Model file for the job. Use its own axes, mm. A direction names the side the tool comes from. Round coordinates to 2 decimals unless told otherwise and drop trailing zeros. Write each loop counter-clockwise with the first axis right and the second up, starting at its lowest first coordinate (ties: lowest second). Pieces come first, ordered by that corner, then holes. Notation, with made-up numbers: (-5.75, 68) - (22.25, 68) arc R35 cw to (22.25, 107) - close; hole circle Ø4 at (20.5, -4). An arc over 180 degrees is marked (long way). Answer as a JSON object with one key per item and string values. Group by question number.
Autodesk Inventor part; units mm, degrees
ref_plane "YZ Plane" through (0, 0, 0) normal (1, 0, 0) x (0, 1, 0)
ref_plane "XZ Plane" through (0, 0, 0) normal (0, 1, 0) x (-1, 0, 0)
ref_plane "XY Plane" through (0, 0, 0) normal (0, 0, 1) x (1, 0, 0)
sketch "Sketch1" plane through (0, 0, 0) normal (0, 1, 0) x (-1, 0, 0)
  line L0 (32, 55) -> (-32, 55)
  line L1 (-32, 55) -> (-32, -55)
  line L2 (-32, -55) -> (32, -55)
  line L3 (32, -55) -> (32, 55)
  line L4 (32, 55) -> (-32, -55) construction
  line L5 (-32, 55) -> (32, -55) construction
  point P0 (0, 0)
  dimension "d0" = 64
  dimension "d1" = 110
extrude "Extrusion1" add sketch "Sketch1" along normal blind 3
sketch "Sketch2" plane through (0, 3, 0) normal (0, 1, 0) x (1, 0, 0)
  line L0 (-32, -55) -> (32, -55)
  line L1 (32, -55) -> (32, 55)
  line L2 (32, 55) -> (-32, 55)
  line L3 (-32, 55) -> (-32, -55)
  line L4 (-32, -55) -> (32, -55)
  line L5 (32, -55) -> (32, 55)
  line L6 (32, 55) -> (-32, 55)
  line L7 (-32, 55) -> (-32, -55)
  line L8 (-32, -55) -> (32, 55) construction
  line L9 (32, -55) -> (-32, 55) construction
  line L10 (-29, -52) -> (29, -52)
  line L11 (29, -52) -> (29, 52)
  line L12 (29, 52) -> (-29, 52)
  line L13 (-29, 52) -> (-29, -52)
  point P0 (0, 0)
  dimension "d4" = 3
  dimension "d5" = 3
  dimension "d6" = 3
  dimension "d7" = 3
extrude "Extrusion2" add sketch "Sketch2" along normal blind 35
sketch "Sketch3" plane through (0, 3, 0) normal (0, 1, 0) x (1, 0, 0)
  line L0 (-23.08, -46) -> (23.08, -46)
  line L1 (23.08, -46) -> (23.08, 46)
  line L2 (23.08, 46) -> (-23.08, 46)
  line L3 (-23.08, 46) -> (-23.08, -46)
  circle A0 centre (-23.08, -46) radius 1.25
  circle A1 centre (23.08, -46) radius 1.25
  circle A2 centre (23.08, 46) radius 1.25
  circle A3 centre (-23.08, 33) radius 1.25
  line L4 (-29, -52) -> (-29, 52)
  line L5 (29, 52) -> (29, -52)
  line L6 (-29, 52) -> (29, 52)
  line L7 (29, -52) -> (-29, -52)
  circle A4 centre (-23.08, -46) radius 3
  circle A5 centre (-23.08, 33) radius 3
  circle A6 centre (23.08, -46) radius 3
  circle A7 centre (23.08, 46) radius 3
  point P0 (0, 0)
  dimension "d15" = 46.16
  dimension "d16" = 92
  dimension "d17" = 2.5
  dimension "d18" = 2.5
  dimension "d19" = 2.5
  dimension "d20" = 2.5
  dimension "d21" = 79
  dimension "d22" = 5.92
  dimension "d23" = 5.92
  dimension "d24" = 6
  dimension "d25" = 6
  dimension "d26" = 6
  dimension "d27" = 6
  dimension "d28" = 6
  dimension "d29" = 6
extrude "Extrusion3" add sketch "Sketch3" along normal blind 6 contours A0 L3 A4 L0 | L0 A4 L3 A0 | A6 L1 A1 L0 | L0 A1 L1 A6 | A5 L3 A3 | L3 A3 A5 | A7 L2 A2 L1 | L1 A2 L2 A7
sketch "Sketch4" plane through (-29, 3, -52) normal (0, 0, 1) x (1, 0, 0)
  line L0 (8.92, 6) -> (2.92, 6)
  line L1 (5.92, 4.5) -> (17.92, 4.5)
  line L2 (17.92, 4.5) -> (17.92, 14.5)
  line L3 (17.92, 14.5) -> (5.92, 14.5)
  line L4 (5.92, 14.5) -> (5.92, 4.5)
  point P0 (29, -3)
  dimension "d33" = 1.5
  dimension "d34" = 10
  dimension "d35" = 12
extrude "Extrusion4" cut sketch "Sketch4" against normal blind 6
sketch "Sketch5" plane through (-29, 3, -52) normal (0, 0, 1) x (1, 0, 0)
  line L0 (17.92, 14.5) -> (17.92, 4.5)
  line L1 (17.92, 4.5) -> (5.92, 4.5)
  line L2 (5.92, 4.5) -> (5.92, 14.5)
  line L3 (5.92, 14.5) -> (17.92, 14.5)
  line L4 (58, 0) -> (0, 0)
  line L5 (58, 0) -> (58, 35)
  line L6 (0, 35) -> (58, 35)
  line L7 (0, 0) -> (0, 35)
  line L8 (24, 31) -> (34, 31)
  line L9 (34, 31) -> (34, 26)
  line L10 (34, 26) -> (24, 26)
  line L11 (24, 26) -> (24, 31)
  line L12 (8.92, 6) -> (2.92, 6)
  point P0 (29, -3)
  dimension "d38" = 20
  dimension "d39" = 5
  dimension "d40" = 10
  dimension "d41" = 24
  dimension "d42" = 24
extrude "Extrusion5" cut sketch "Sketch5" against normal blind 6 contours L8 L9 L10 L11
sketch "Sketch7" plane through (0, 0, 0) normal (0, -1, 0) x (1, 0, 0)
  line L0 (29, 52) -> (-29, 52)
  line L1 (-29, 52) -> (-29, -52)
  line L2 (-29, -52) -> (29, -52)
  line L3 (29, -52) -> (29, 52)
  line L4 (29, 52) -> (-29, 52)
  line L5 (32, -55) -> (-32, -55)
  line L6 (-32, -55) -> (-32, 55)
  line L7 (-32, 55) -> (32, 55)
  line L8 (32, 55) -> (32, -55)
  line L9 (32, 55) -> (32, -55)
  circle A0 centre (32, 55) radius 4.2426
  point P0 (0, 0)
extrude "Extrusion6" add sketch "Sketch7" against normal blind 38 contours A0 L7 L8 | A0 L8 L7
sketch "Sketch8" plane through (0, 38, 0) normal (0, 1, 0) x (1, 0, 0)
  arc A0 (27.7574, -55) -> (32, -50.7574) centre (32, -55) ccw
  circle A1 centre (32, -55) radius 1.65
  point P0 (0, 0)
  dimension "d47" = 3.3
extrude "Extrusion7" cut sketch "Sketch8" against normal blind 15
mirror "Mirror1" about plane through (0, 0, 0) normal (1, 0, 0) of "Extrusion6", "Extrusion7"
mirror "Mirror2" about plane through (0, 0, 0) normal (0, 0, 1) of "Extrusion6", "Extrusion7", "Mirror1"
sketch "Sketch9" plane through (-29, 3, 52) normal (1, 0, 0) x (0, 0, -1)
  line L0 (88, 6) -> (82, 6)
  circle A0 centre (82, 20) radius 6
  line L1 (85, 6) -> (85, 35)
  line L2 (0, 35) -> (104, 35)
  line L3 (85, 6) -> (114, 6) construction
  point P0 (52, -3)
  dimension "d50" = 12
  dimension "d51" = 14
  dimension "d52" = 90
  dimension "d53" = 3
extrude "Extrusion8" cut sketch "Sketch9" against normal through all
sketch "Sketch10" plane through (27.7574, 0, -55) normal (0, 0, -1) x (-1, 0, 0)
  line L0 (21.7574, 0) -> (33.7574, 0)
  line L1 (33.7574, 0) -> (33.7574, 4)
  line L2 (33.7574, 4) -> (21.7574, 4)
  line L3 (21.7574, 4) -> (21.7574, 0)
  line L4 (55.5147, 0) -> (55.5147, 38)
  line L5 (0, 38) -> (0, 0)
  point P0 (27.7574, 0)
  dimension "d56" = 4
  dimension "d57" = 12
  dimension "d58" = 21.7574
  dimension "d59" = 21.7574
extrude "Extrusion9" add sketch "Sketch10" along normal blind 14
chamfer "Chamfer1" distance 2 angle 45 3 edges at (6, 2, -55) (-6, 2, -55) (0, 4, -55)
sketch "Sketch11" plane through (-6, 4, -69) normal (0, 1, 0) x (1, 0, 0)
  line L0 (12, -12) -> (0, -12)
  line L1 (12, -12) -> (12, 0)
  line L2 (0, 0) -> (12, 0)
  line L3 (0, -12) -> (0, 0)
  circle A0 centre (6, -6) radius 2.6
  point P0 (6, -69)
  dimension "d65" = 5.2
  dimension "d66" = 6
  dimension "d67" = 6
extrude "Extrusion10" cut sketch "Sketch11" against normal through all contours A0
mirror "Mirror3" about plane through (0, 0, 0) normal (0, 0, 1) of "Extrusion9", "Extrusion10"
chamfer "Chamfer2" distance 2 angle 45 3 edges at (-6, 2, 55) (0, 4, 55) (6, 2, 55)
equation "\"d4\" = d5"
equation "\"d6\" = d5"
equation "\"d7\" = d5"
equation "\"d22\" = d23"
equation "\"d24\" = d25"
equation "\"d27\" = d26"
equation "\"d28\" = d26"
equation "\"d29\" = d26"
equation "\"d41\" = d42"
equation "\"d58\" = d59"
equation "\"d67\" = d66"
properties part number "Podstawa"
(1) Slice it at C-C (y = 15.5). Write the cut outline in (x, z).
(2) Drill centre lines: line 1 (Z direction, x = 23, y = 6.5); line 2 (X direction, y = 4.3, z = 46); line 3 (Z direction, x = 0, y = 2.4). Where is each one in solid material? Low to high. Write a range as from..to.
(3) 3-axis set-ups, long thin cutter, end or side, ignore diameter. For faces 1 (the flat face through (0, 4, -60)), 2 (the flat face through (6, 2, -63)), 3 (the cylindrical face through (-20.22, 5.96, -32.1)), 4 (the flat face through (-23.08, 13, -53)): which of +Z, -Z, +X, -X, +Y, -Y reach the whole face in a straight line?
(4) Slice it at A-A (z = -63). Write the cut outline in (x, y), then the cut area to 3 significant figures.
(5) Slice it at D-D (z = -10). Write the cut outline in (x, y).
(6) Flat gauge pins, fed straight in: pin 1 (4 mm diameter, centred on x = -24.5, y = 33, fed in from +Z); pin 2 (4 mm diameter, centred on x = -23.08, z = 46, fed in from +Y); pin 3 (4 mm diameter, centred on y = 11, z = -8.5, fed in from +X). Where does each tip first touch, or does it go through?
(7) Slice it at B-B (x = -15). Write the cut outline in (y, z).
(8) Pull direction Z, two halves, no side cores. Call faces 5 (the cylindrical face through (-35, 19, 58)), 6 (the cylindrical face through (-21.89, 5.96, 46.38)), 7 (the flat face through (0, 29, -53)): pulls with the +Z half, pulls with the -Z half, needs draft (parallel to the pull), parting line crosses it, or undercut.
Answer:
{
 "1": {"outline": "(-32, -50.76) arc R4.24 ccw (long way) to (-27.76, -55) - (-23.08, -55) - (-23.08, -52) - (-29, -52) - (-29, 52) - (29, 52) - (29, -52) - (-11.08, -52) - (-11.08, -55) - (27.76, -55) arc R4.24 ccw (long way) to (32, -50.76) - (32, 50.76) arc R4.24 ccw (long way) to (27.76, 55) - (-27.76, 55) arc R4.24 ccw (long way) to (-32, 50.76) - close"},
 "2": {"line 1": "-55..-52, -49..-47.25, -44.75..-43, 43..44.75, 47.25..49, 52..55", "line 2": "-32..-29, -26.08..-24.33, -21.83..-20.08, 20.08..21.83, 24.33..26.08, 29..32", "line 3": "-69..-65.6, -60.4..60.4, 65.6..69"},
 "3": {"face 1": "-Z, +Y", "face 2": "-Z, +Y, -Y", "face 3": "+Y", "face 4": "-Z"},
 "4": {"outline": "(-6, 0) - (-2.6, 0) - (-2.6, 4) - (-6, 4) - close; (2.6, 0) - (6, 0) - (6, 4) - (2.6, 4) - close", "area": "27.2 mm²"},
 "5": {"outline": "(-32, 0) - (32, 0) - (32, 38) - (29, 38) - (29, 3) - (-29, 3) - (-29, 38) - (-32, 38) - close"},
 "6": {"pin 1": "z = 55", "pin 2": "y = 9", "pin 3": "x = 32"},
 "7": {"outline": "(0, -55) - (7.5, -55) - (7.5, -52) - (3, -52) - (3, 52) - (38, 52) - (38, 55) - (0, 55) - close; (17.5, -55) - (38, -55) - (38, -52) - (17.5, -52) - close"},
 "8": {"face 5": "undercut", "face 6": "undercut", "face 7": "needs draft"}
}
